The listing builds one solid part. Answer for the finished solid, in the listing's coordinates (mm). A direction names the side the tool comes from. Give positions to 0.01 mm unless a question says otherwise; leave off trailing zeros. Order: outer loops, then holes, each group sorted by start corner. A loop starts at its lowest first (then second) coordinate and runs counter-clockwise, first axis right, second up. Notation, with made-up numbers: (33.25, 37.25) - (61.25, 37.25) arc R16 cw to (61.25, 59.25) - close; hole circle Ø2 at (0, -34.5). An arc over 180 degrees is marked (long way). Answer in a Markdown table with one row per item.
from build123d import *

# Parameters (mm, degrees)
EXTRUDE_1_DEPTH     = 25
SHELL_1_T           = -2.2
SKETCH_2_W          = 20.6
SKETCH_2_H          = 20.6
CUT_EXTRUDE_1_DEPTH = 5
SKETCH_3_R          = 3
CUT_EXTRUDE_2_DEPTH = 451


with BuildPart() as part:
    # Эскиз1 → Бобышка-Вытянуть1 (new body)
    with BuildSketch(Plane.XY):
        with BuildLine():
            Line((-260.93597277, 123.115577889), (-260.93597277, -226.884422111))
            ThreePointArc((-260.93597277, -226.884422111), (-238.968981359, -279.9174307), (-185.93597277, -301.884422111))
            Line((-185.93597277, -301.884422111), (114.06402723, -301.884422111))
            ThreePointArc((114.06402723, -301.884422111), (167.097035819, -279.9174307), (189.06402723, -226.884422111))
            Line((189.06402723, -226.884422111), (189.06402723, 123.115577889))
            Line((189.06402723, 123.115577889), (164.06402723, 123.115577889))
            Line((164.06402723, 123.115577889), (164.06402723, -226.884422111))
            ThreePointArc((164.06402723, -226.884422111), (149.419366289, -262.23976117), (114.06402723, -276.884422111))
            Line((114.06402723, -276.884422111), (-185.93597277, -276.884422111))
            ThreePointArc((-185.93597277, -276.884422111), (-221.291311829, -262.23976117), (-235.93597277, -226.884422111))
            Line((-235.93597277, -226.884422111), (-235.93597277, 123.115577889))
            Line((-235.93597277, 123.115577889), (-260.93597277, 123.115577889))
        make_face()
    extrude(amount=EXTRUDE_1_DEPTH)

    # Оболочка1
    shell_1_openings = [part.faces().sort_by_distance(p)[0] for p in [
        (-248.43597277, 123.115577889, 12.5),
    ]]
    offset(amount=SHELL_1_T, openings=shell_1_openings, kind=Kind.INTERSECTION)

    # Эскиз2 → Вырез-Вытянуть1 (cut)
    with BuildSketch(Plane(origin=(0, 123.115577889, 0), x_dir=(1, 0, 0), z_dir=(0, 1, 0))):
        with Locations((176.56402723, -12.5)):
            Rectangle(SKETCH_2_W, SKETCH_2_H)
    extrude(amount=-CUT_EXTRUDE_1_DEPTH, mode=Mode.SUBTRACT)

    # Эскиз3 → Вырез-Вытянуть2 (cut, through all)
    with BuildSketch(Plane.ZY.offset(260.93597277)):
        with Locations(Location((12.5, 108.115577889, 0), (0, 0, 270))):  # turned: the seam where the file's is
            Circle(SKETCH_3_R)
        with Locations(Location((12.5, 88.115577889, 0), (0, 0, 270))):  # turned: the seam where the file's is
            Circle(SKETCH_3_R)
    extrude(amount=-CUT_EXTRUDE_2_DEPTH, mode=Mode.SUBTRACT)


solid = part.part
Item 1: Find section B-B on x = 144.5. Write down the section's boundary in (y, z).
Answer block:
| item | result |
|---|---|
| outline | (-295.43, 0) - (-266.55, 0) - (-266.55, 25) - (-295.43, 25) - close; hole (-293.02, 2.2) - (-269.29, 2.2) - (-269.29, 22.8) - (-293.02, 22.8) - close |
Item 2: Find section C-C on y = -252.5. Write down the section's boundary in (x, z).
Answer block:
| item | result |
|---|---|
| outline | (-256.43, 0) - (-228.88, 0) - (-228.88, 25) - (-256.43, 25) - close; (157, 0) - (184.55, 0) - (184.55, 25) - (157, 25) - close; hole (-254.08, 2.2) - (-231.42, 2.2) - (-231.42, 22.8) - (-254.08, 22.8) - close; hole (159.55, 2.2) - (182.21, 2.2) - (182.21, 22.8) - (159.55, 22.8) - close |
Item 3: Consider line 1 (X direction, y = -207.5, z = 5.25); line 2 (Y direction, x = -90.5, z = 16.75); line 3 (X direction, y = -229, z = 20.5). Determine where each line is inside the solid, lowest interval first.
Answer block:
| item | result |
|---|---|
| line 1 | -260.94 to -258.74, -238.14 to -235.94, 164.06 to 166.26, 186.86 to 189.06 |
| line 2 | -301.88 to -299.68, -279.08 to -276.88 |
| line 3 | -260.91 to -258.71, -238.09 to -235.89, 164.02 to 166.22, 186.83 to 189.03 |
Item 4: Determine the mould class of faces 1 (the face through (166.264, -49, 12)), 2 (the face through (-258.736, -49, 12)), 3 (the face through (-34, -276.884, 12)), 4 (the face through (-70.3, -277.3, 0)) for opening direction Z: pulls with the +Z half, pulls with the -Z half, needs draft (parallel to the pull), parting line crosses it, or undercut.
Answer block:
| item | result |
|---|---|
| face 1 | undercut |
| face 2 | undercut |
| face 3 | needs draft |
| face 4 | pulls with the -Z half |
Item 5: Each of these flat-tipped pins is pushed along its axis until it touches: P1, Ø1, axis at x = 13.5, z = 10, coming from the +Y side; P2, Ø1.5, axis at y = -241, z = 3, coming from the +X side; P3, Ø5, axis at y = -254, z = 20, coming from the +X side. Where does it stop, or does it pass through?
Answer block:
| item | result |
|---|---|
| P1 | y = -276.88 |
| P2 | x = 187.86 |
| P3 | x = 184.91 |
Item 6: Which of the six approach directions +Z, -Z, +X, -X, +Y, -Y give full straight-line access (tool end or side, diameter ignored) to faces 5 (the face through (-222.44, -264.2, 12.36)), 6 (the face through (186.864, -54, 12)), 7 (the face through (149.806, -261.849, 12.325))?
Answer block:
| item | result |
|---|---|
| face 5 | none |
| face 6 | +Y |
| face 7 | +Z, -Z, +Y |
Item 7: Find section D-D on x = 67. Write down the section's boundary in (y, z).
Answer block:
| item | result |
|---|---|
| outline | (-301.88, 0) - (-276.88, 0) - (-276.88, 25) - (-301.88, 25) - close; hole (-299.68, 2.2) - (-279.08, 2.2) - (-279.08, 22.8) - (-299.68, 22.8) - close |
Item 8: Find section A-A on y = -80. Write down the section's boundary in (x, z).
Answer block:
| item | result |
|---|---|
| outline | (-260.94, 0) - (-235.94, 0) - (-235.94, 25) - (-260.94, 25) - close; (164.06, 0) - (189.06, 0) - (189.06, 25) - (164.06, 25) - close; hole (-258.74, 2.2) - (-238.14, 2.2) - (-238.14, 22.8) - (-258.74, 22.8) - close; hole (166.26, 2.2) - (186.86, 2.2) - (186.86, 22.8) - (166.26, 22.8) - close |
